Verification items for the finished model (mm, model axes). Face numbers are marked on the shaded views. A direction names the side the tool comes from. Round coordinates to 2 decimals unless told otherwise and drop trailing zeros. Order: outer loops, then holes, each group sorted by start corner. A loop starts at its lowest first (then second) coordinate and runs counter-clockwise, first axis right, second up. Notation, with made-up numbers: M 72,-21 L 120,-21 A17 cw 120,1 Z; hole C 25,53.25 d1. An arc over 180 degrees is marked long. Write item = value, one per line. Start each with the question number.
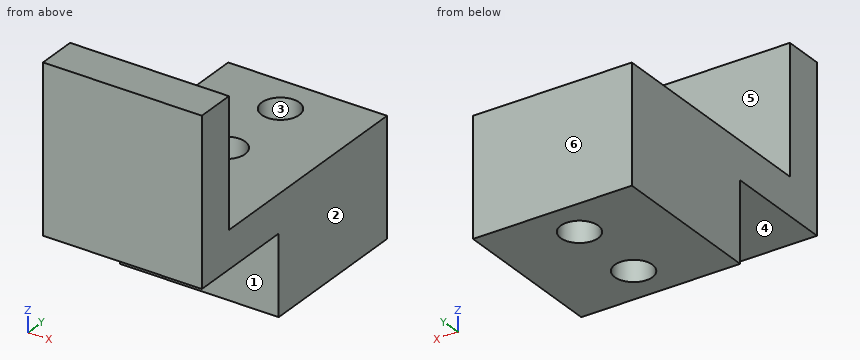
from build123d import *

# Parameters (mm, degrees)
BOSS_EXTRUDE1_DEPTH = 6.35
SKETCH2_R           = 1.5
CUT_EXTRUDE1_DEPTH  = 10.3472


with BuildPart() as part:
    # Sketch1 → Boss-Extrude1 (new body, symmetric)
    with BuildSketch(Plane(origin=(0, 0, 0), x_dir=(0, 0, -1), z_dir=(1, 0, 0))):
        Polygon((0, 12.7), (0, 0), (-6.35, 0), (-6.35, -9.017), (-19.5072, -9.017), (-19.5072, -5.842), (-9.3472, -5.842), (-9.3472, 12.7), align=None)
    extrude(amount=BOSS_EXTRUDE1_DEPTH, both=True)

    # Sketch2 → Cut-Extrude1 (cut, through all)
    with BuildSketch(Plane.XY.offset(9.3472)):
        with Locations((0, 9.525)):
            Circle(SKETCH2_R)
        with Locations((0, 3.175)):
            Circle(SKETCH2_R)
    extrude(amount=-CUT_EXTRUDE1_DEPTH, mode=Mode.SUBTRACT)


solid = part.part
1) Scan lines: probe 1 along Y at (x, z) = (0, 7.25) (3 decimals); probe 2 along Y at (x, z) = (0, 6) (3 decimals); probe 3 along Z at (x, y) = (5.25, 9.75). Record each from-to range of solid material in increasing order.
2) Gauge pin test, flat ends, axial feed: P1, Ø4, axis at x = 0, y = 9.525, coming from the +Z side; P2, Ø3, axis at x = 1.5, z = 15, coming from the +Y side; P3, Ø5, axis at x = 1.5, y = 2, coming from the -Z side; P4, Ø5, axis at x = -3, z = 3, coming from the -Y side. Record the tip position at first contact, or that the pin passes through.
3) Cross-section at B-B, the plane y = 5. Enter the section's corners in (x, z).
4) Access from +Z, -Z, +X, -X, +Y, -Y to the whole of each face (thin tool, end or side, straight path). Record for the marked faces 4, 5 and 6.
5) Cross-section at A-A, the plane x = 0. Enter the section's corners in (y, z) (3 decimals), then the cut area to 3 significant figures.
6) Release check for a two-part mould opening along Y. For the marked faces 1, 2 and 3 record: pulls with the +Y half, pulls with the -Y half, needs draft (parallel to the pull), parting line crosses it, or undercut.
7) Cross-section at C-C, the plane x = -3.75. Enter the section's corners in (y, z), then the cut area to 3 significant figures.
8) Cross-section at D-D, the plane z = 10. Enter the section's corners in (x, y).
Geometry results:
q1.probe_1 = -9.017 to 1.675, 4.675 to 8.025, 11.025 to 12.7
q1.probe_2 = 0 to 1.675, 4.675 to 8.025, 11.025 to 12.7
q1.probe_3 = 0 to 9.35
q2.P1 = 9.35
q2.P2 = -5.84
q2.P3 = 0
q2.P4 = 0
q3.outline = M -6.35,0 L 6.35,0 L 6.35,9.35 L -6.35,9.35 Z
q4.face_4 = -Z, +X, -X, -Y
q4.face_5 = +Z, +X, -X, +Y
q4.face_6 = +Z, -Z, +X, -X, +Y
q5.outline = M -9.017,6.35 L 0,6.35 L 0,0 L 1.675,0 L 1.675,9.347 L -5.842,9.347 L -5.842,19.507 L -9.017,19.507 Z; M 4.675,0 L 8.025,0 L 8.025,9.347 L 4.675,9.347 Z; M 11.025,0 L 12.7,0 L 12.7,9.347 L 11.025,9.347 Z
q5.area = 122 mm^2
q6.face_1 = pulls with the -Y half
q6.face_2 = needs draft
q6.face_3 = undercut
q7.outline = M -9.02,6.35 L 0,6.35 L 0,0 L 12.7,0 L 12.7,9.35 L -5.84,9.35 L -5.84,19.51 L -9.02,19.51 Z
q7.area = 178 mm^2
q8.outline = M -6.35,-9.02 L 6.35,-9.02 L 6.35,-5.84 L -6.35,-5.84 Z
